For this review, use the dimensioned drawing (mm, ordinates from the lowest corner) and the shaded views. A direction names the side the tool comes from. Coordinates: 2 decimals unless noted, no trailing zeros. Write each loop counter-clockwise with the first axis right and the second up, starting at its lowest first coordinate (ties: lowest second). Pieces come first, ordered by that corner, then holes.
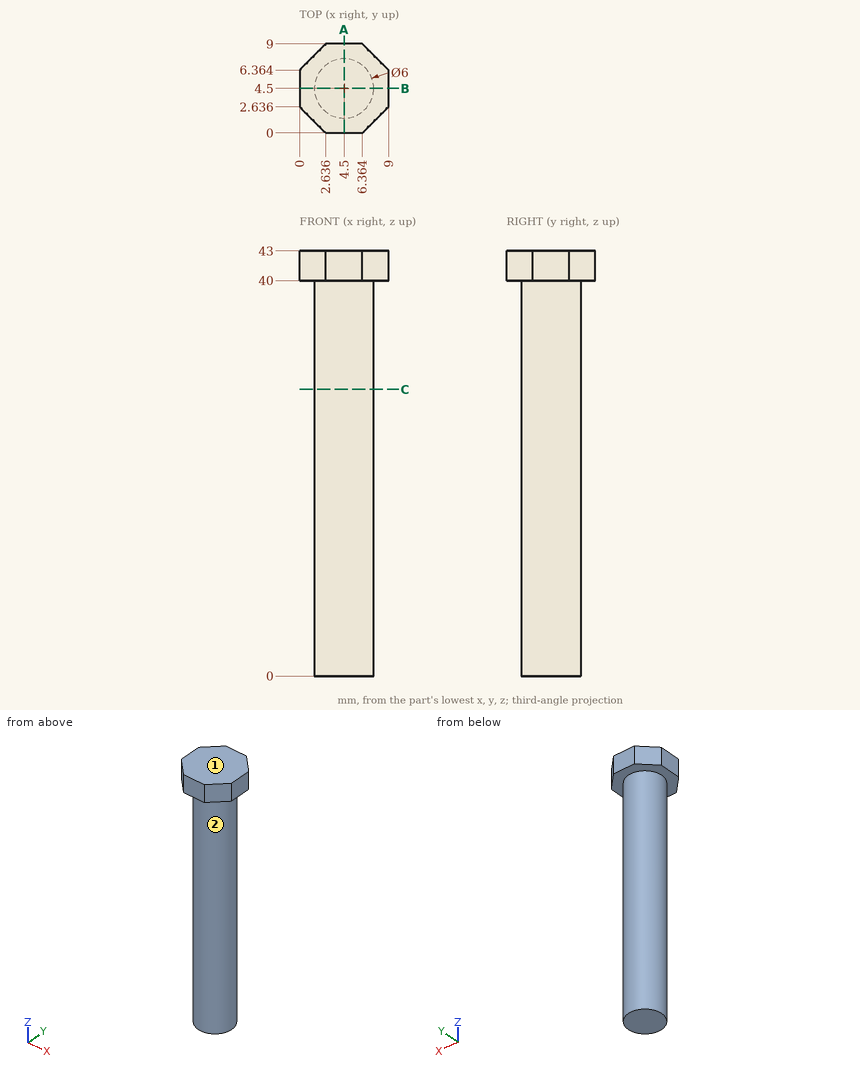
Item 1: To check wall thickness, follow line 1 along Z through (x, y) = (1, 5.5); line 2 along X through (y, z) = (2, 28.5); line 3 along X through (y, z) = (1.75, 25.5). State the ranges of each line that lie inside material, in increasing order.
Solved:
line 1: z = 40 to 43
line 2: x = 2.84 to 6.16
line 3: x = 3.3 to 5.7
Item 2: Take a section at A-A, the plane x = 4.5. Write out the cut boundary in (y, z).
Solved:
outline: (0, 40) - (1.5, 40) - (1.5, 0) - (7.5, 0) - (7.5, 40) - (9, 40) - (9, 43) - (0, 43) - close
Item 3: Take a section at C-C, the plane z = 29. Write out the cut boundary in (x, y), plus the area to 3 significant figures.
Solved:
outline: circle Ø6 at (4.5, 4.5)
area: 28.3 mm2
Item 4: Machinability: for the marked faces 1 and 2, which of the approach directions +Z, -Z, +X, -X, +Y, -Y give a long, thin tool a straight path to every point of the face, cutting with its end or side? Answer none if there is none.
Solved:
face 1: +Z, +X, -X, +Y, -Y
face 2: -Z
Item 5: For pin 1 (1 mm diameter, centred on x = 2, z = 22, fed in from -Y); pin 2 (3 mm diameter, centred on x = 2.5, z = 24, fed in from +Y), all flat-tipped, find the tip position at first contact; note any pin that passes through.
Solved:
pin 1: stops at y = 2.26
pin 2: stops at y = 7.46
